from build123d import *

# Parameters (mm, degrees)
BOSS_EXTRUDE1_DEPTH = 50
SKETCH2_R           = 11.05
SKETCH2_R_2         = 2
CUT_EXTRUDE1_DEPTH  = 3
CUT_EXTRUDE2_DEPTH  = 50
BOSS_EXTRUDE2_DEPTH = 2
BOSS_EXTRUDE3_DEPTH = 2
CHAMFER1_SIZE       = 5


with BuildPart() as part:
    # Sketch1 → Boss-Extrude1 (new body)
    with BuildSketch(Plane.XY):
        Polygon((0, 0), (0, 51), (2, 51), (2, 2), (53, 2), (53, 0), align=None)
    extrude(amount=BOSS_EXTRUDE1_DEPTH)

    # Sketch2 → Cut-Extrude1 (cut, through all)
    with BuildSketch(Plane(origin=(2, 0, 0), x_dir=(0, 0, -1), z_dir=(1, 0, 0))):
        with Locations((-25, 30)):
            Circle(SKETCH2_R)
        with Locations((-40.5, 45.640445987)):
            Circle(SKETCH2_R_2)
        with Locations((-9.5, 45.5)):
            Circle(SKETCH2_R_2)
        with Locations((-40.5, 14.5)):
            Circle(SKETCH2_R_2)
        with Locations((-9.5, 14.5)):
            Circle(SKETCH2_R_2)
    extrude(amount=-CUT_EXTRUDE1_DEPTH, mode=Mode.SUBTRACT)

    # Sketch3 → Cut-Extrude2 (cut)
    with BuildSketch(Plane(origin=(0, 2, 0), x_dir=(1, 0, 0), z_dir=(0, 1, 0))):
        with BuildLine():
            Line((12.455251015, -12.1), (42.544748985, -12.1))
            ThreePointArc((42.544748985, -12.1), (44.644629774, -9.977624237), (42.5, -7.900476833))
            Line((42.5, -7.900476833), (12.5, -7.900476833))
            ThreePointArc((12.5, -7.900476833), (10.355370226, -9.977624237), (12.455251015, -12.1))
        make_face()
        with BuildLine():
            Line((12.5, -42.099523167), (42.5, -42.099523167))
            ThreePointArc((42.5, -42.099523167), (44.644629774, -40.022375763), (42.544748985, -37.9))
            Line((42.544748985, -37.9), (12.455251015, -37.9))
            ThreePointArc((12.455251015, -37.9), (10.355370226, -40.022375763), (12.5, -42.099523167))
        make_face()
    extrude(amount=-CUT_EXTRUDE2_DEPTH, mode=Mode.SUBTRACT)

    # Sketch5 → Boss-Extrude2 (add)
    with BuildSketch(Plane.XY.offset(50)):
        Polygon((2, 22), (2, 4), (4, 2), (15, 2), align=None)
    extrude(amount=-BOSS_EXTRUDE2_DEPTH)

    # Sketch6 → Boss-Extrude3 (add)
    with BuildSketch(Plane(origin=(0, 0, 0), x_dir=(-1, 0, 0), z_dir=(0, 0, -1))):
        Polygon((-4, 2), (-2, 4), (-2, 22), (-15, 2), align=None)
    extrude(amount=-BOSS_EXTRUDE3_DEPTH)

    # Chamfer1
    chamfer1_edges = [part.edges().sort_by_distance(p)[0] for p in [
        (1, 51, 50),
        (1, 51, 0),
        (53, 1, 50),
        (53, 1, 0),
    ]]
    chamfer(chamfer1_edges, length=CHAMFER1_SIZE)


solid = part.part
The listing builds one solid part. Answer for the finished solid, in the listing's coordinates (mm). A direction names the side the tool comes from. Coordinates: 2 decimals unless noted, no trailing zeros. Order: outer loops, then holes, each group sorted by start corner. A loop starts at its lowest first (then second) coordinate and runs counter-clockwise, first axis right, second up. Notation, with made-up numbers: (31.25, 11) -> (57.25, 11) arc R21 cw to (57.25, 34) -> close; hole circle Ø11 at (48.25, 20). An arc over 180 degrees is marked (long way). Answer in a Markdown table with one row per item. Add a question column.
Item 1: Find section B-B (x = 19). Write down the section's boundary in (y, z).
Item 2: Find section D-D (y = 5). Write down the section's boundary in (x, z), then the cut area to 3 significant figures.
Item 3: Find the intervals of material crossed by L1, parallel to Y at x = 1.5, z = 9.5; L2, parallel to Y at x = 0.45, z = 40.5; L3, parallel to Y at x = 1, z = 25, in increasing order. Write a range as from..to.
Item 4: Find section C-C (y = 30). Write down the section's boundary in (x, z).
Item 5: Each of these flat-tipped pins is pushed along its axis until it touches: P1, Ø14.5, axis at y = 17.5, z = 18.5, coming from the +X side; P2, Ø12, axis at x = 18, z = 20.5, coming from the +Y side. Where does it stop, or does it pass through?
Item 6: Find section A-A (z = 25). Write down the section's boundary in (x, y).
Item 7: Which of the six approach directions +Z, -Z, +X, -X, +Y, -Y give full straight-line access (tool end or side, diameter ignored) to faces 1 (the face through (10.355, 1.014, 39.976)), 2 (the face through (1.014, 43.726, 8.577)), 3 (the face through (6, 8, 2))?
Item 8: Determine the mould class of faces 4 (the face through (10, 9, 50)), 5 (the face through (1.01, 33.32, 14.46)), 6 (the face through (27, 0, 25)), 7 (the face through (27, 1, 12.1)) for opening direction Z: +Z half, -Z half, draft (parallel to the pull), parting line (faces both ways), or undercut.
Result set:
| question | item | result |
|---|---|---|
| 1 | outline | (0, 0) -> (2, 0) -> (2, 7.9) -> (0, 7.9) -> close; (0, 12.1) -> (2, 12.1) -> (2, 37.9) -> (0, 37.9) -> close; (0, 42.1) -> (2, 42.1) -> (2, 50) -> (0, 50) -> close |
| 2 | outline | (0, 0) -> (13.05, 0) -> (13.05, 2) -> (2, 2) -> (2, 48) -> (13.05, 48) -> (13.05, 50) -> (0, 50) -> close |
| 2 | area | 144 mm² |
| 3 | L1 | y = 0..12.5, 16.5..43.5, 47.5..51 |
| 3 | L2 | y = 0..12.5, 16.5..43.64, 47.64..51 |
| 3 | L3 | y = 0..18.95, 41.05..51 |
| 4 | outline | (0, 0) -> (2, 0) -> (2, 13.95) -> (0, 13.95) -> close; (0, 36.05) -> (2, 36.05) -> (2, 50) -> (0, 50) -> close |
| 5 | P1 | stops at x = 2 |
| 5 | P2 | stops at y = 2 |
| 6 | outline | (0, 0) -> (53, 0) -> (53, 2) -> (2, 2) -> (2, 18.95) -> (0, 18.95) -> close; (0, 41.05) -> (2, 41.05) -> (2, 51) -> (0, 51) -> close |
| 7 | face 1 | +Y, -Y |
| 7 | face 2 | +X, -X |
| 7 | face 3 | +X, +Y |
| 8 | face 4 | +Z half |
| 8 | face 5 | undercut |
| 8 | face 6 | draft |
| 8 | face 7 | undercut |
